from build123d import *

# Parameters (mm, degrees)
F1_DEPTH = 48.514
F2_W     = 15.8159341663
F2_H     = 83.4212787449
F3_DEPTH = 25.4
F5_DEPTH = 25.4


with BuildPart() as f1:
    # F0 (on Right) → F1 (new body)
    with BuildSketch(Plane.YZ):
        Polygon((-41.7106375098, 22.4834308028), (-41.7106375098, -47.6028472185), (41.7106412351, -48.2230819762), (41.7106412351, 22.4834308028), align=None)
    extrude(amount=F1_DEPTH)

    # F2 (on face) → F3 (cut)
    with BuildSketch(Plane.XY.offset(22.4834308028)):
        with Locations((23.2587223873, 1.8626e-06)):
            Rectangle(F2_W, F2_H)
    extrude(amount=-F3_DEPTH, mode=Mode.SUBTRACT)

    # F4 (on face) → F5 (cut)
    with BuildSketch(Plane(origin=(0, -0.3562117937, -47.9103161593), x_dir=(1, 0, 0), z_dir=(0, -0.0074347651, -0.9999723618))):
        Polygon((48.514, -14.4669022411), (48.514, -0.3562235017), (0, 0), (0, -0.3562235017), (0, -14.4669022411), align=None)
    extrude(amount=-F5_DEPTH, mode=Mode.SUBTRACT)


solid = f1.part
Work out the finished part from the listing and answer in its coordinate system (mm). A direction names the side the tool comes from. Coordinates: 2 decimals unless noted, no trailing zeros. Write each loop counter-clockwise with the first axis right and the second up, starting at its lowest first coordinate (ties: lowest second). Pieces come first, ordered by that corner, then holes. Notation, with made-up numbers: M -30.75,12 L -10.75,12 A22 ccw -10.75,51 Z; hole C 31,8.25 d1. An arc over 180 degrees is marked long. Answer as CSV lines item,"result". Start each with the question number.
Item 1: Determine the mould class of faces 1 (the face through (40, 1, 22.483)), 2 (the face through (48.514, -1, -12)), 3 (the face through (0, -1, -12)), 4 (the face through (23, 1, -2.917)) for opening direction X: released by +X, released by -X, zero draft, split by the parting line, or undercut.
Item 2: Section A-A on z = 17 is taken. Write down the section's boundary in (x, y).
Item 3: A tool of negligible diameter and unlimited length cuts with its end or side. For faces 5 (the face through (15.351, -1, 10)), 6 (the face through (24, 41.711, -13)), from which of +Z, -Z, +X, -X, +Y, -Y can it reach the whole face along a straight path? Write none if from no direction.
Item 4: Flat-ended cylindrical pins translate along their axes: P1, Ø8, axis at x = 23, y = 14, coming from the +Z side; P2, Ø10, axis at x = 40, y = -16, coming from the -Z side. Find the tip coordinate at first contact, or state that the pin passes through.
Item 5: Consider L1, parallel to X at y = 3.5, z = 4; L2, parallel to Z at x = 13.5, y = 2.5; L3, parallel to Y at x = 9, z = -43.5. Determine where each line is inside the solid, lowest interval first.
Item 6: Section C-C on x = 33 is taken. Write down the section's boundary in (y, z).
Item 7: Section D-D on z = -24 is taken. Write down the section's boundary in (x, y).
Item 8: Section B-B on y = -25.5 is taken. Write down the section's boundary in (x, z), and give its area (3 significant figures).
Checks:
1,face 1,"zero draft"
1,face 2,"released by +X"
1,face 3,"released by -X"
1,face 4,"undercut"
2,outline,"M 0,-41.71 L 15.35,-41.71 L 15.35,41.71 L 0,41.71 Z; M 31.17,-41.71 L 48.51,-41.71 L 48.51,41.71 L 31.17,41.71 Z"
3,face 5,"+Z, +Y, -Y"
3,face 6,"+Z, -Z, +X, -X, +Y"
4,P1,"stops at z = -2.92"
4,P2,"stops at z = -47.83"
5,L1,"x = 0 to 15.35, 31.17 to 48.51"
5,L2,"z = -22.53 to 22.48"
5,L3,"y = -41.71 to -0.26, 14.14 to 41.71"
6,outline,"M -41.71,-47.6 L -0.11,-47.91 L 0.07,-22.51 L 14.3,-22.62 L 14.11,-48.02 L 41.71,-48.22 L 41.71,22.48 L -41.71,22.48 Z"
7,outline,"M 0,-41.71 L 48.51,-41.71 L 48.51,0.18 L 0,-0.18 Z; M 0,14.29 L 48.51,14.29 L 48.51,41.71 L 0,41.71 Z"
8,outline,"M 0,-47.72 L 48.51,-47.72 L 48.51,22.48 L 31.17,22.48 L 31.17,-2.92 L 15.35,-2.92 L 15.35,22.48 L 0,22.48 Z"
8,area,"3,000 mm²"
